Verification items for the finished model (mm, model axes). A direction names the side the tool comes from. Round coordinates to 2 decimals unless told otherwise and drop trailing zeros. Order: outer loops, then holes, each group sorted by start corner. A loop starts at its lowest first (then second) coordinate and runs counter-clockwise, first axis right, second up. Notation, with made-up numbers: (41.25, 64) -> (45.25, 64) arc R13 cw to (45.25, 75) -> close; hole circle Ø2 at (-1, -26). An arc over 180 degrees is marked (long way). Answer in a Markdown table with one row per item. Add a question column.
```python
from build123d import *

# Parameters (mm, degrees)
EXTRUDE_1_DEPTH     = 40
SKETCH_2_R          = 15
CUT_EXTRUDE_1_DEPTH = 35
SKETCH_3_R          = 3
CUT_EXTRUDE_2_DEPTH = 12


with BuildPart() as part:
    # 草图1 → 凸台-拉伸1 (new body)
    with BuildSketch(Plane.XY):
        with BuildLine():
            Line((20, 25), (-20, 25))
            Line((-20, 25), (-20, 0))
            ThreePointArc((-20, 0), (0, -20), (20, 0))
            Line((20, 0), (20, 25))
        make_face()
    extrude(amount=EXTRUDE_1_DEPTH)

    # 草图2 → 切除-拉伸1 (cut)
    with BuildSketch(Plane.XY.offset(40)):
        Circle(SKETCH_2_R)
    extrude(amount=-CUT_EXTRUDE_1_DEPTH, mode=Mode.SUBTRACT)

    # 草图3 → 切除-拉伸2 (cut)
    with BuildSketch(Plane(origin=(0, 25, 0), x_dir=(1, 0, 0), z_dir=(0, 1, 0))):
        with Locations(Location((11.153964198, -7.5, 0), (0, 0, 270))):
            Circle(SKETCH_3_R)
        with Locations(Location((-11.153964198, -7.5, 0), (0, 0, 90))):
            Circle(SKETCH_3_R)
        with Locations(Location((11.153964198, -32.5, 0), (0, 0, 270))):
            Circle(SKETCH_3_R)
        with Locations(Location((-11.153964198, -32.5, 0), (0, 0, 90))):
            Circle(SKETCH_3_R)
    extrude(amount=-CUT_EXTRUDE_2_DEPTH, mode=Mode.SUBTRACT)


solid = part.part
```
1) Tool access check on faces 1 (the face through (-11, 13, 33)), 2 (the face through (-14.985, 0.66, 22.745)), 3 (the face through (0, 25, 20)). Record the directions out of +Z, -Z, +X, -X, +Y, -Y that give a thin tool (end or side, any length) a straight path to the whole face; none if there is none.
2) Depth check by flat-ended pin: P1, Ø1.8, axis at x = -11, z = 6, coming from the +Y side; P2, Ø5, axis at x = -5.5, z = 33, coming from the -Y side; P3, Ø6, axis at x = -10, y = 4.5, coming from the +Z side. Enter the tip coordinate at first touch or a pass-through.
3) Cross-section at A-A, the plane z = 17. Record the boundary of the cut face in (x, y).
4) Cross-section at B-B, the plane y = 20.5. Record the boundary of the cut face in (x, z).
5) Cross-section at D-D, the plane z = 7.5. Record the boundary of the cut face in (x, y).
6) Thickness scan on L1, parallel to X at y = 17, z = 7.5; L2, parallel to Y at x = 0, z = 26.5; L3, parallel to X at y = 21, z = 7. Record the ranges inside material, lowest first. Write a range as [from, to].
7) Draft check along Z on faces 4 (the face through (-9, 13, 40)), 5 (the face through (11.286, 19.084, 29.503)), 6 (the face through (0, -20, 20)). Enter one of: +Z half, -Z half, draft (parallel to the pull), parting line (faces both ways), or undercut.
8) Cross-section at C-C, the plane x = 0. Record the boundary of the cut face in (y, z), and give its area (3 significant figures).
Results below:
| question | item | result |
|---|---|---|
| 1 | face 1 | +Y |
| 1 | face 2 | +Z |
| 1 | face 3 | +Z, -Z, +X, -X, +Y |
| 2 | P1 | y = 13 |
| 2 | P2 | y = -19.77 |
| 2 | P3 | z = 5 |
| 3 | outline | (-20, 0) arc R20 ccw to (20, 0) -> (20, 25) -> (-20, 25) -> close; hole circle Ø30 at (0, 0) |
| 4 | outline | (-20, 0) -> (20, 0) -> (20, 40) -> (-20, 40) -> close; hole circle Ø6 at (-11.15, 7.5); hole circle Ø6 at (-11.15, 32.5); hole circle Ø6 at (11.15, 7.5); hole circle Ø6 at (11.15, 32.5) |
| 5 | outline | (-20, 0) arc R20 ccw to (20, 0) -> (20, 25) -> (14.15, 25) -> (14.15, 13) -> (8.15, 13) -> (8.15, 25) -> (-8.15, 25) -> (-8.15, 13) -> (-14.15, 13) -> (-14.15, 25) -> (-20, 25) -> close; hole circle Ø30 at (0, 0) |
| 6 | L1 | [-20, -14.15], [-8.15, 8.15], [14.15, 20] |
| 6 | L2 | [-20, -15], [15, 25] |
| 6 | L3 | [-20, -14.11], [-8.2, 8.2], [14.11, 20] |
| 7 | face 4 | +Z half |
| 7 | face 5 | undercut |
| 7 | face 6 | draft |
| 8 | outline | (-20, 0) -> (25, 0) -> (25, 40) -> (15, 40) -> (15, 5) -> (-15, 5) -> (-15, 40) -> (-20, 40) -> close |
| 8 | area | 750 mm² |
